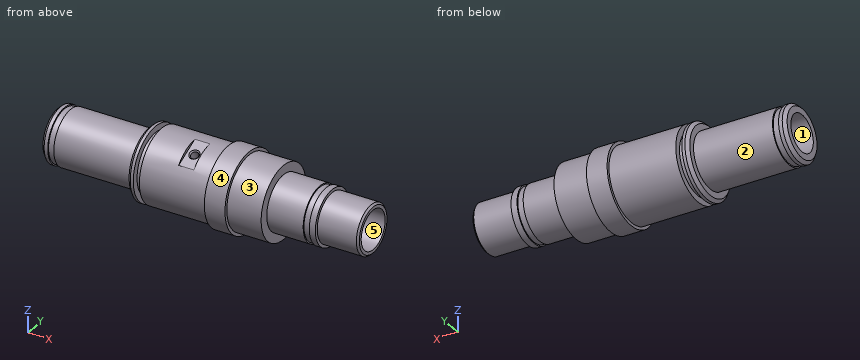
Autodesk Inventor part; units mm, degrees
ref_plane "YZ Plane" through (0, 0, 0) normal (1, 0, 0) x (0, 1, 0)
ref_plane "XZ Plane" through (0, 0, 0) normal (0, 1, 0) x (-1, 0, 0)
ref_plane "XY Plane" through (0, 0, 0) normal (0, 0, 1) x (1, 0, 0)
sketch "Sketch2" plane through (0, 0, 0) normal (0, 0, 1) x (1, 0, 0)
  line L0 (0, 4) -> (0.5, 4.5)
  line L1 (0, 4) -> (0, 3)
  line L2 (0.5, 4.5) -> (1.1, 4.5)
  line L3 (1.1, 4.5) -> (1.1, 4.3)
  line L4 (1.1, 4.3) -> (2.1, 4.3)
  line L5 (2.1, 4.3) -> (2.1, 4.5)
  line L6 (2.1, 4.5) -> (15.1, 4.5)
  line L7 (15.1, 4.5) -> (15.1, 5.5)
  line L8 (15.1, 5.5) -> (15.6, 6)
  line L9 (0, 3) -> (20, 3)
  line L10 (20, 3) -> (20.2, 3.2)
  line L11 (44.15, 4.5) -> (44.15, 4.3)
  line L12 (44.15, 4.3) -> (43.15, 4.3)
  line L13 (43.15, 4.3) -> (43.15, 4.5)
  line L14 (0, 0) -> (27.0854, 0) construction
  line L15 (15.6, 6) -> (16.1, 6)
  line L16 (16.1, 6) -> (16.1, 5)
  line L17 (16.1, 5) -> (17.1, 5)
  line L18 (17.1, 5) -> (17.1, 6)
  line L19 (31.9, 6) -> (31.5, 6)
  line L20 (31.5, 6) -> (31.5, 6.5)
  line L21 (31.5, 6.5) -> (28.1, 6.5)
  line L22 (28.1, 6.5) -> (28.1, 6)
  line L23 (17.1, 6) -> (28.1, 6)
  line L24 (20.2, 3.2) -> (43.9, 3.2)
  line L25 (44.15, 4.5) -> (45.15, 4.5)
  line L26 (43.15, 4.5) -> (37.9, 4.5)
  line L27 (37.15, 6) -> (31.9, 6)
  line L28 (43.9, 3.2) -> (49.9, 3.2)
  line L29 (49.9, 4) -> (45.15, 4)
  line L30 (45.15, 4) -> (45.15, 4.5)
  line L31 (49.9, 3.2) -> (51.9, 3.2)
  line L32 (51.9, 3.2) -> (51.9, 4)
  line L33 (51.9, 4) -> (49.9, 4)
  line L34 (37.9, 4.5) -> (37.15, 4.5)
  line L35 (37.15, 4.5) -> (37.15, 6)
  point P0 (1.1, 4.4)
  point P1 (15.85, 6)
  point P2 (16.6, 5)
  dimension "d3" = 4
  dimension "d8" = 1
  dimension "d9" = 0.5
  dimension "d10" = 0.5
  dimension "d11" = 0.2
  dimension "d12" = 1
  dimension "d13" = 13
  dimension "d14" = 1
  dimension "d15" = 20
  dimension "d26" = 0.2
  dimension "d27" = 0.2
  dimension "d29" = 0.5
  dimension "d30" = 0.5
  dimension "d36" = 1.1
  dimension "d37" = 4.5
  dimension "d38" = 3
  dimension "d39" = 0.5
  dimension "d40" = 1
  dimension "d41" = 1
  dimension "d60" = 0.4
  dimension "d61" = 0.5
  dimension "d62" = 3.4
  dimension "d63" = 11
  dimension "d65" = 1
  dimension "d66" = 5.25
  dimension "d83" = 6
  dimension "d84" = 0.8
  dimension "d85" = 2
  dimension "d86" = 0.75
revolve "Revolution1" add sketch "Sketch2" angle 360 about axis through (0, 0, 0) along (1, 0, 0)
thread "Thread1"
ref_plane "Work Plane1" through (51.1424, -20, -139.2633) normal (0, 1, 0) x (-1, 0, 0)
sketch "Sketch4" plane through (17.1, 0, 0) normal (-1, 0, 0) x (0, 0, 1)
  circle A0 centre (0, 0) radius 6
  point P0 (0, 6)
  point P1 (6, 0)
  point P2 (0, -6.0107)
  point P3 (-6.0435, 0)
ref_plane "Work Plane2" through (22.6, -2.6349, 5.3905) normal (0, 0.4392, -0.8984) x (1, 0, 0)
ref_plane "Work Plane3" through (25.4, -2.6349, 5.3905) normal (0, 0.4392, -0.8984) x (1, 0, 0)
sketch "Sketch7" plane through (22.6, -2.6349, 5.3905) normal (0, 0.4392, -0.8984) x (1, 0, 0)
  line L0 (2.6, 5) -> (0.1, 5)
  line L1 (0.1, 5) -> (0.1, -5)
  line L2 (0.1, -5) -> (2.6, -5)
  line L3 (2.6, -5) -> (2.6, 5)
  line L4 (2.6, 5) -> (0.1, -5) construction
  line L5 (0.1, 5) -> (2.6, -5) construction
  line L6 (-22.6, -4) -> (-22.6, 4) construction
  point P0 (-22.6, 0)
  point P1 (1.35, 0)
  dimension "d68" = 2.5
  dimension "d69" = 10
  dimension "d70" = 23.95
extrude "Extrusion3" cut sketch "Sketch7" along normal blind 0.5
hole "Hole2" at (23.95, -2.6349, 5.3905) direction (0, 0.4392, -0.8984) diameter 1.221 depth 5.3 tip angle 118
chamfer "Chamfer2" distance 0.2 angle 45 1 edges at (23.95, -1.8669, 5.2094)
chamfer "Chamfer3" distance 0.3 angle 45 1 edges at (51.9, -4, 0)
properties part number "nakrętka"
Here's how the part is built. I have some questions about the finished solid (model axes, mm). Face numbers are marked on the shaded views. A direction names the side the tool comes from. Round coordinates to 2 decimals unless told otherwise and drop trailing zeros. Write each loop counter-clockwise with the first axis right and the second up, starting at its lowest first coordinate (ties: lowest second). Pieces come first, ordered by that corner, then holes.
1. If we mould it in two halves opening along Y, with no side actions, what happens to the marked faces 4 and 5? For each: released by +Y, released by -Y, zero draft, split by the parting line, or undercut.
2. Suppose I cut it at B-B (x = 22). List the corners of the cut face in (y, z) for me, and give its area (3 significant figures).
3. Will these pins go through, and if not, where does the flat tip stop? pin 1 Ø1.7 at (y, z) = (-3, 5) entering from +X; pin 2 Ø2.5 at (y, z) = (0, 0) entering from +X; pin 3 Ø1.5 at (x, y) = (15, -2.5) entering from +Z; pin 4 Ø2.5 at (y, z) = (-1.5, 5.5) entering from -X.
4. I need wall thicknesses on L1, parallel to X at y = 5.5, z = 0.25; L2, parallel to Z at x = 11.5, y = 0; L3, parallel to X at y = -3.5, z = 3. Which ranges of each line are inside material? Lowest first, please.
5. For the marked faces 1, 2 and 3, which set-ups out of +Z, -Z, +X, -X, +Y, -Y let a thin tool reach every point of the face, with its end or its side?
6. Suppose I cut it at A-A (x = 47). List the corners of the cut face in (y, z) for me, and give its area (3 significant figures).
Answer sheet:
1. face 4: split by the parting line
1. face 5: undercut
2. outline: circle Ø12 at (0, 0); hole circle Ø6.4 at (0, 0)
2. area: 80.9 mm2
3. pin 1: stops at x = 37.15
3. pin 2: passes through
3. pin 3: stops at z = 5.64
3. pin 4: stops at x = 0.45
4. L1: x = 15.11 to 16.1, 17.1 to 37.15
4. L2: z = -4.5 to -3, 3 to 4.5
4. L3: x = 15.1 to 37.15
5. face 1: +X, -X
5. face 2: -X
5. face 3: +X
6. outline: circle Ø8 at (0, 0); hole circle Ø6.4 at (0, 0)
6. area: 18.1 mm2
